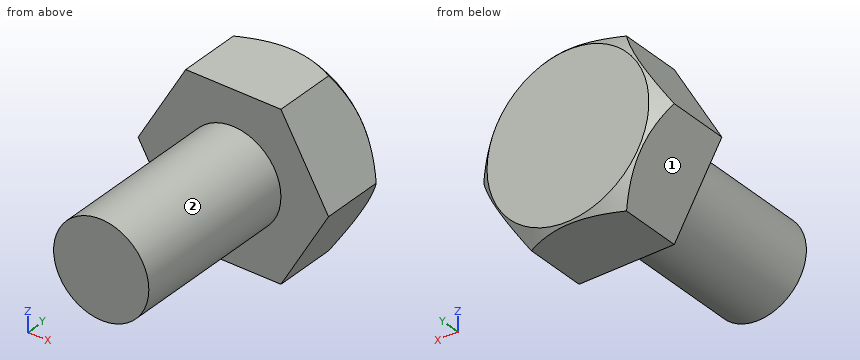
```python
from build123d import *

# Parameters (mm, degrees)
SKETCH1_R           = 2.5
BOSS_EXTRUDE1_DEPTH = 9
BOSS_EXTRUDE4_DEPTH = 4
SKETCH5_OUTSIDE_W   = 23.71
SKETCH5_OUTSIDE_H   = 22.37
SKETCH5_OUTSIDE_R   = 4.25
CUT_EXTRUDE1_DEPTH  = 4
CUT_EXTRUDE1_TAPER  = 45


with BuildPart() as part:
    # Sketch1 → Boss-Extrude1 (new body)
    with BuildSketch(Plane(origin=(0, 0, 0), x_dir=(1, 0, 0), z_dir=(0, 1, 0))):
        Circle(SKETCH1_R)
    extrude(amount=BOSS_EXTRUDE1_DEPTH)

    # Sketch3 → Boss-Extrude4 (add)
    with BuildSketch(Plane(origin=(0, 9, 0), x_dir=(1, 0, 0), z_dir=(0, 1, 0))):
        Polygon((5, 0), (2.5, 4.330127019), (-2.5, 4.330127019), (-5, 0), (-2.5, -4.330127019), (2.5, -4.330127019), align=None)
    extrude(amount=BOSS_EXTRUDE4_DEPTH)

    # Sketch5 outside → Cut-Extrude1 (cut)
    with BuildSketch(Plane(origin=(0, 13, 0), x_dir=(1, 0, 0), z_dir=(0, 1, 0))):
        Rectangle(SKETCH5_OUTSIDE_W, SKETCH5_OUTSIDE_H)
        Circle(SKETCH5_OUTSIDE_R, mode=Mode.SUBTRACT)
    extrude(amount=-CUT_EXTRUDE1_DEPTH, taper=CUT_EXTRUDE1_TAPER, mode=Mode.SUBTRACT)


solid = part.part
```
Source: CAD feature listing. Evaluate the final solid. Frame: model axes, mm. Face numbers are marked on the shaded views. A direction names the side the tool comes from. Coordinates: 2 decimals unless noted, no trailing zeros. Loops run counter-clockwise (first coordinate to the right, second up) from the corner with the lowest first, then second, coordinate; pieces in that order, holes last. Notation, with made-up numbers: (-22, -31.75) -> (-18, -31.75) arc R29 cw to (-18, 4.25) -> close; hole circle Ø9 at (-30, -26). An arc over 180 degrees is marked (long way). One line per item, written item: value. Start each with the question number.
Q1. Set-up query: the marked faces 1 and 2. Return all of +Z, -Z, +X, -X, +Y, -Y with unobstructed straight access to the full face (end or side cutting, diameter ignored); none if empty.
Q2. Line query: line 1 along Y through (x, z) = (-3.5, 1.25); line 2 along X through (y, z) = (8.25, 2); line 3 along Z through (x, y) = (4, 11.25). Output: solid intervals per line, ascending.
Q3. Section query A-A, the plane x = 0. Return the cut outline in (y, z).
Q4. Section query B-B, the plane y = 5.5. Return the cut outline in (x, z).
Q5. Contact query for flat-ended pins moving along their axis: P1, Ø1.5, axis at y = 3.5, z = -1.5, coming from the -X side; P2, Ø3, axis at x = 2, y = 6.5, coming from the +Z side; P3, Ø4.5, axis at x = -0.5, z = -0.5, coming from the -Y side; P4, Ø2, axis at y = 5.5, z = 0, coming from the +X side. Output: stop coordinate, or through.
Results:
1. face 1: -Z, -X, +Y, -Y
1. face 2: -Y
2. line 1: 9 to 13
2. line 2: -1.5 to 1.5
2. line 3: -1.73 to 1.73
3. outline: (0, -2.5) -> (9, -2.5) -> (9, -4.33) -> (12.92, -4.33) -> (13, -4.25) -> (13, 4.25) -> (12.92, 4.33) -> (9, 4.33) -> (9, 2.5) -> (0, 2.5) -> close
4. outline: circle Ø5 at (0, 0)
5. P1: x = -2.38
5. P2: z = 2.45
5. P3: y = 0
5. P4: x = 2.5
